Study the drawing (mm; zero at the part's minimum x, y, z) and answer. A direction names the side the tool comes from. Coordinates: 2 decimals unless noted, no trailing zeros. Order: outer loops, then holes, each group sorted by start corner. A loop starts at its lowest first (then second) coordinate and runs counter-clockwise, first axis right, second up. Notation, with made-up numbers: (82, 33.5) -> (95, 33.5) arc R23 ccw to (95, 63.5) -> close; hole circle Ø8 at (48, 18.25). An arc over 180 degrees is marked (long way). Answer as CSV lines item,"result". Start each with the question number.
Item 1: Section A-A (z = 8.75) is taken. Write down the section's boundary in (x, y).
Item 2: Each of these flat-tipped pins is pushed along its axis until it touches: pin 1 Ø5 at (x, y) = (5, 6) entering from +Z; pin 2 Ø1.8 at (x, y) = (57, 5) entering from -Z. Where does it stop, or does it pass through?
Item 3: For a pull along X with two mould halves and no side action, classify the marked faces 1, 2 and 3 as pulls with the +X half, pulls with the -X half, needs draft (parallel to the pull), parting line crosses it, or undercut.
Item 4: Straight lines are drawn through the part: L1, parallel to X at y = 6, z = 7; L2, parallel to X at y = 0.5, z = 9; L3, parallel to Y at x = 57, z = 8.3. For each, find the intervals that lie inside material, in ascending order.
Item 5: Section D-D (y = 1.75) is taken. Write down the section's boundary in (x, z).
Item 6: Section C-C (x = 57) is taken. Write down the section's boundary in (y, z).
Item 7: Section B-B (y = 5) is taken. Write down the section's boundary in (x, z).
Item 8: Which of the six approach directions +Z, -Z, +X, -X, +Y, -Y give full straight-line access (tool end or side, diameter ignored) to the marked faces 4 and 5?
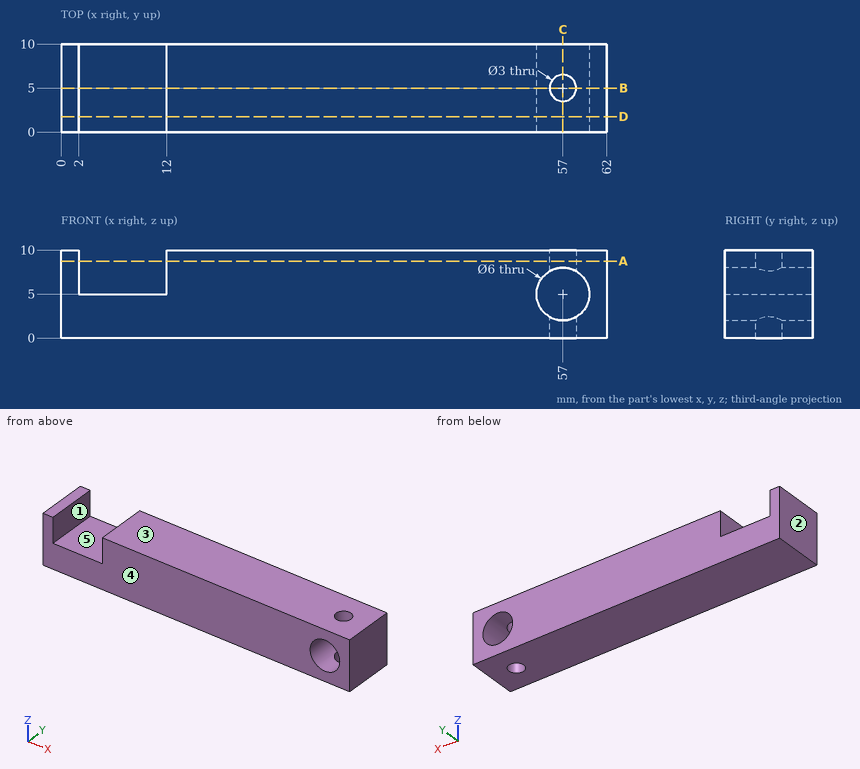
Checked values:
1,outline,"(0, 0) -> (2, 0) -> (2, 10) -> (0, 10) -> close; (12, 0) -> (62, 0) -> (62, 10) -> (12, 10) -> close; hole circle Ø3 at (57, 5)"
2,pin 1,"stops at z = 5"
2,pin 2,"passes through"
3,face 1,"undercut"
3,face 2,"pulls with the -X half"
3,face 3,"needs draft"
4,L1,"x = 0 to 2, 12 to 54.76, 59.24 to 62"
4,L2,"x = 0 to 2, 12 to 62"
4,L3,"y = 0 to 3.5, 6.5 to 10"
5,outline,"(0, 0) -> (62, 0) -> (62, 10) -> (12, 10) -> (12, 5) -> (2, 5) -> (2, 10) -> (0, 10) -> close; hole circle Ø6 at (57, 5)"
6,outline,"(0, 0) -> (3.5, 0) -> (3.5, 2) -> (0, 2) -> close; (0, 8) -> (3.5, 8) -> (3.5, 10) -> (0, 10) -> close; (6.5, 0) -> (10, 0) -> (10, 2) -> (6.5, 2) -> close; (6.5, 8) -> (10, 8) -> (10, 10) -> (6.5, 10) -> close"
7,outline,"(0, 0) -> (55.5, 0) -> (55.5, 2.4) arc R3 cw to (55.5, 7.6) -> (55.5, 10) -> (12, 10) -> (12, 5) -> (2, 5) -> (2, 10) -> (0, 10) -> close; (58.5, 0) -> (62, 0) -> (62, 10) -> (58.5, 10) -> (58.5, 7.6) arc R3 cw to (58.5, 2.4) -> close"
8,face 4,"+Z, -Z, +X, -X, -Y"
8,face 5,"+Z, +Y, -Y"
